Source: CAD feature listing. Evaluate the final solid. Frame: model axes, mm. A direction names the side the tool comes from. Coordinates: 2 decimals unless noted, no trailing zeros. Order: outer loops, then holes, each group sorted by start corner. A loop starts at its lowest first (then second) coordinate and runs counter-clockwise, first axis right, second up. Notation, with made-up numbers: (56.5, 47.5) -> (91.5, 47.5) arc R19 cw to (91.5, 55.5) -> close; hole circle Ø7 at (-33, 26). An arc over 180 degrees is marked (long way). Put each result on its own line as item: value.
from build123d import *

# Parameters (mm, degrees)
SKETCH1_W                 = 28.448
SKETCH1_H                 = 25.4
BOSS_EXTRUDE1_DEPTH       = 63.5
SKETCH2_W                 = 8.636
SKETCH2_H                 = 31.75
CUT_EXTRUDE1_DEPTH        = 70.855079815
SKETCH3_R                 = 3.175
CUT_EXTRUDE3_DEPTH        = 71.730677248
F_6_32_TAPPED_HOLE1_D     = 2.7051
F_6_32_TAPPED_HOLE1_DEPTH = 6.35
F_6_32_TAPPED_HOLE1_TIP   = 0.81269403
F_6_32_TAPPED_HOLE2_D     = 2.7051
F_6_32_TAPPED_HOLE2_DEPTH = 6.35
F_6_32_TAPPED_HOLE2_TIP   = 0.81269403
F_6_32_TAPPED_HOLE3_D     = 2.7051


with BuildPart() as part:
    # Sketch1 → Boss-Extrude1 (new body)
    with BuildSketch(Plane.XY):
        Rectangle(SKETCH1_W, SKETCH1_H)
    extrude(amount=BOSS_EXTRUDE1_DEPTH)

    # Sketch2 → Cut-Extrude1 (cut, through all)
    with BuildSketch(Plane(origin=(0, 12.7, 0), x_dir=(1, 0, 0), z_dir=(0, 1, 0))):
        with Locations((0, -15.875)):
            Rectangle(SKETCH2_W, SKETCH2_H)
    extrude(amount=-CUT_EXTRUDE1_DEPTH, mode=Mode.SUBTRACT)

    # Sketch3 → Cut-Extrude3 (cut, through all)
    with BuildSketch(Plane.ZY.offset(14.224)):
        with Locations((15.875, 0)):
            Circle(SKETCH3_R)
    extrude(amount=-CUT_EXTRUDE3_DEPTH, mode=Mode.SUBTRACT)

    # #6-32 Tapped Hole1
    with Locations(Plane.ZY.offset(14.224)):
        with Locations((5.715, 0), (53.975, 0)):
            Hole(F_6_32_TAPPED_HOLE1_D / 2, depth=F_6_32_TAPPED_HOLE1_DEPTH)
            with Locations((0, 0, -(F_6_32_TAPPED_HOLE1_DEPTH + F_6_32_TAPPED_HOLE1_TIP / 2))):  # 118° drill point
                Cone(0, F_6_32_TAPPED_HOLE1_D / 2, F_6_32_TAPPED_HOLE1_TIP, mode=Mode.SUBTRACT)

    # #6-32 Tapped Hole2
    with Locations(Plane(origin=(14.224, 0, 0), x_dir=(0, 0, -1), z_dir=(1, 0, 0))):
        with Locations((-53.975, 0), (-5.715, 0)):
            Hole(F_6_32_TAPPED_HOLE2_D / 2, depth=F_6_32_TAPPED_HOLE2_DEPTH)
            with Locations((0, 0, -(F_6_32_TAPPED_HOLE2_DEPTH + F_6_32_TAPPED_HOLE2_TIP / 2))):  # 118° drill point
                Cone(0, F_6_32_TAPPED_HOLE2_D / 2, F_6_32_TAPPED_HOLE2_TIP, mode=Mode.SUBTRACT)

    # #6-32 Tapped Hole3 (through all)
    with Locations(Plane(origin=(0, 0, 31.75), x_dir=(-1, 0, 0), z_dir=(0, 0, -1))):
        with Locations((0, 0)):
            Hole(F_6_32_TAPPED_HOLE3_D / 2)


solid = part.part
1. Cut plane C-C on y = -6. Output: boundary loops of the cut face in (x, z), plus the area to 3 significant figures.
Numbers:
outline: (-14.22, 0) -> (-4.32, 0) -> (-4.32, 31.75) -> (4.32, 31.75) -> (4.32, 0) -> (14.22, 0) -> (14.22, 63.5) -> (-14.22, 63.5) -> close
area: 1,530 mm2
2. Set-up query: faces 5 (the cylindrical face through (11.005, 0.059, 52.624)), 6 (the flat face through (4.318, 0, 20)), 7 (the flat face through (0, 3, 63.5)), 8 (the flat face through (9, 0, 0)), 9 (the cylindrical face through (-11.005, 0.406, 52.685)). Return all of +Z, -Z, +X, -X, +Y, -Y with unobstructed straight access to the full face (end or side cutting, diameter ignored); none if empty.
Numbers:
face 5: +X
face 6: -Z, +Y, -Y
face 7: +Z, +X, -X, +Y, -Y
face 8: -Z, +X, -X, +Y, -Y
face 9: -X
3. Cut plane B-B on x = 0. Output: boundary loops of the cut face in (y, z).
Numbers:
outline: (-12.7, 31.75) -> (-1.35, 31.75) -> (-1.35, 63.5) -> (-12.7, 63.5) -> close; (1.35, 31.75) -> (12.7, 31.75) -> (12.7, 63.5) -> (1.35, 63.5) -> close
4. Ray query, line 1 along X through (y, z) = (-3.5, 17.5); line 2 along Y through (x, z) = (0, 47.5); line 3 along X through (y, z) = (1, 47.5). Return the intervals inside material, ascending.
Numbers:
line 1: x = -14.22 to -4.32, 4.32 to 14.22
line 2: y = -12.7 to -1.35, 1.35 to 12.7
line 3: x = -14.22 to -0.91, 0.91 to 14.22
5. First-contact query: pin 1 (2.5 mm diameter, centred on y = 0, z = 53.975, fed in from +X); pin 2 (2 mm diameter, centred on y = 0, z = 53.975, fed in from -X). Flat tips, straight axial feed; report the tip coordinate or a pass-through.
Numbers:
pin 1: stops at x = 7.81
pin 2: stops at x = -7.66
6. Cut plane D-D on x = 12. Output: boundary loops of the cut face in (y, z) (3 decimals).
Numbers:
outline: (-12.7, 0) -> (12.7, 0) -> (12.7, 63.5) -> (-12.7, 63.5) -> close; hole circle Ø6.35 at (0, 15.875); hole circle Ø2.705 at (0, 5.715); hole circle Ø2.705 at (0, 53.975)
7. Cut plane A-A on z = 25. Output: boundary loops of the cut face in (x, y).
Numbers:
outline: (-14.22, -12.7) -> (-4.32, -12.7) -> (-4.32, 12.7) -> (-14.22, 12.7) -> close; (4.32, -12.7) -> (14.22, -12.7) -> (14.22, 12.7) -> (4.32, 12.7) -> close
8. Pull-direction query (Z, two-part tool) for faces 1 (the cylindrical face through (9.202, 0.954, 18.903)), 2 (the flat face through (0, -12.7, 38)), 3 (the conical face through (7.202, 0.071, 53.751)), 4 (the flat face through (-9, 0, 0)); classes: pulls with the +Z half, pulls with the -Z half, needs draft (parallel to the pull), parting line crosses it, or undercut.
Numbers:
face 1: undercut
face 2: needs draft
face 3: undercut
face 4: pulls with the -Z half
